```python
from build123d import *

# Parameters (mm, degrees)
SKETCH_1_W          = 5
SKETCH_1_H          = 1
SKETCH_1_W_2        = 3
EXTRUDE_1_DEPTH     = 1
SKETCH_1_3_W        = 3
SKETCH_1_3_H        = 1
EXTRUDE_2_DEPTH     = 2
SKETCH_1_4_W        = 5
SKETCH_1_4_H        = 1
EXTRUDE_3_DEPTH     = 4
SKETCH_2_W          = 1
SKETCH_2_H          = 1
CUT_EXTRUDE_1_DEPTH = 4


with BuildPart() as part:
    # Sketch 1 → Extrude 1 (new body)
    with BuildSketch(Plane(origin=(0, 0, 0), x_dir=(1, 0, 0), z_dir=(0, 1, 0))):
        with Locations((3.5, 3.5)):
            Rectangle(SKETCH_1_W, SKETCH_1_H)
        Polygon((3, 0), (4, 0), (6, 2), (6, 3), (1, 3), (1, 4), (0, 4), (0, 1), (3, 1), align=None)
        with Locations((1.5, 0.5)):
            Rectangle(SKETCH_1_W_2, SKETCH_1_H)
    extrude(amount=EXTRUDE_1_DEPTH)

    # Sketch 1_3 → Extrude 2 (add)
    with BuildSketch(Plane(origin=(0, 0, 0), x_dir=(1, 0, 0), z_dir=(0, 1, 0))):
        with Locations((1.5, 0.5)):
            Rectangle(SKETCH_1_3_W, SKETCH_1_3_H)
    extrude(amount=EXTRUDE_2_DEPTH)

    # Sketch 1_4 → Extrude 3 (add)
    with BuildSketch(Plane(origin=(0, 0, 0), x_dir=(1, 0, 0), z_dir=(0, 1, 0))):
        with Locations((3.5, 3.5)):
            Rectangle(SKETCH_1_4_W, SKETCH_1_4_H)
    extrude(amount=EXTRUDE_3_DEPTH)

    # Sketch 2 → Cut-Extrude 1 (cut)
    with BuildSketch(Plane.XY.offset(-3)):
        with Locations((4.5, 2.5)):
            Rectangle(SKETCH_2_W, SKETCH_2_H)
        Polygon((1, 4), (3, 4), (1, 1), align=None)
    extrude(amount=-CUT_EXTRUDE_1_DEPTH, mode=Mode.SUBTRACT)


solid = part.part
```
The model under review builds one solid part; all positions refer to its coordinate system, in mm. A direction names the side the tool comes from. Give positions to 0.01 mm unless a question says otherwise; leave off trailing zeros. Write each loop counter-clockwise with the first axis right and the second up, starting at its lowest first coordinate (ties: lowest second). Pieces come first, ordered by that corner, then holes. Notation, with made-up numbers: M -18.5,-27 L 35.5,-27 A8 ccw 35.5,-16 Z; hole C 65.5,-38 d6. An arc over 180 degrees is marked long. Write each question's results on one line, items separated by ' | '. Start each with the question number.
1. For faces 4 (the flat face through (4.5, 3, -3.5)), 5 (the flat face through (3, 1.5, -0.5)), 6 (the flat face through (3, 2, -3)), 7 (the flat face through (2, 2.5, -3.5)), list the 3-axis set-ups (+Z, -Z, +X, -X, +Y, -Y) from which the entire face can be reached by the end or side of a thin tool; tool diameter is ignored.
2. We need section B-B (x = 4.25). Write out the cut boundary in (y, z), and give its area (3 significant figures).
3. Insertion check: pin 1 Ø0.8 at (y, z) = (1.5, -0.5) entering from +X; pin 2 Ø1.1 at (y, z) = (2.5, -3.5) entering from -X; pin 3 Ø1.2 at (x, z) = (4.5, -2) entering from +Y. Each pin has a flat end and moves straight along its axis. Give the tip position at first contact, or say it passes through.
4. For probe 1 along Y at (x, z) = (3.1, -2.25); probe 2 along Z at (x, y) = (5.3, 2.75); probe 3 along X at (y, z) = (2.55, -3.45), list the stretches that pass through material, from the lowest coordinate up. Write a range as [from, to].
5. We need section D-D (z = -0.45). Write out the cut boundary in (x, y), and give its area (3 significant figures).
6. Mouldability with a two-part tool opening along Y and no side actions: class faces 1 (the flat face through (1.5, 2, -0.5)), 2 (the flat face through (4.5, 2, -3.5)), 3 (the flat face through (0, 0.8, -1.6)) as released by +Y, released by -Y, zero draft, split by the parting line, or undercut.
7. We need section C-C (z = -3.25). Write out the cut boundary in (x, y).
8. We need section A-A (y = 1.15). Write out the cut boundary in (x, z), and give its area (3 significant figures).
Results found:
1) face 4: +Z, -Z | face 5: +Z, +X, +Y | face 6: +X, -X, +Y | face 7: -Z, -X, +Y
2) outline: M 0,-4 L 2,-4 L 2,-3 L 1,-3 L 1,-0.25 L 0,-0.25 Z; M 3,-4 L 4,-4 L 4,-3 L 3,-3 Z | area: 5.75 mm^2
3) pin 1: stops at x = 3 | pin 2: stops at x = 1.63 | pin 3: stops at y = 1
4) probe 1: y = [0, 1] | probe 2: z = [-4, -3] | probe 3: x = [2.03, 4], [5, 6]
5) outline: M 0,0 L 4.45,0 L 4.45,1 L 3,1 L 3,2 L 0,2 Z | area: 7.45 mm^2
6) face 1: released by +Y | face 2: undercut | face 3: zero draft
7) outline: M 0,0 L 6,0 L 6,4 L 3,4 L 1,1 L 0,1 Z; hole M 4,2 L 5,2 L 5,3 L 4,3 Z
8) outline: M 0,-1 L 3,-1 L 3,0 L 0,0 Z; M 1.1,-4 L 6,-4 L 6,-3 L 1.1,-3 Z | area: 7.90 mm^2
